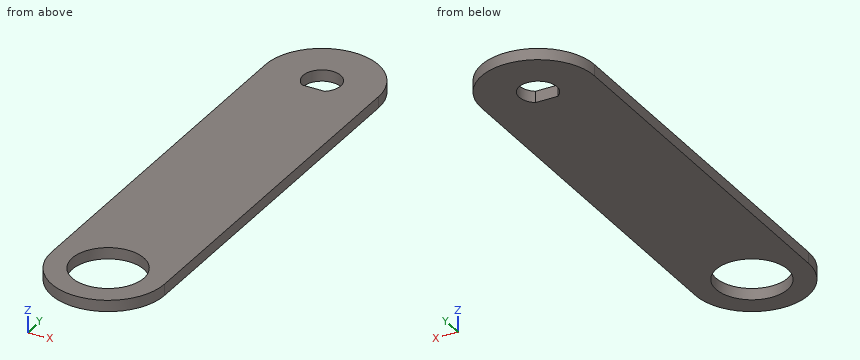
```python
from build123d import *

# Parameters (mm, degrees)
SKETCH_1_R      = 9.5
EXTRUDE_1_DEPTH = 3


with BuildPart() as part:
    # 草图1 → 凸台-拉伸1 (new body)
    with BuildSketch(Plane.XY):
        with BuildLine():
            Line((-15, 0), (-15, -100))
            ThreePointArc((-15, -100), (0, -115), (15, -100))
            Line((15, -100), (15, 0))
            ThreePointArc((15, 0), (0, 15), (-15, 0))
        make_face()
        with Locations((0, -100)):
            Circle(SKETCH_1_R, mode=Mode.SUBTRACT)
        with BuildLine():
            Line((0, -4), (3, -4))
            ThreePointArc((3, -4), (0, 5), (-3, -4))
            Line((-3, -4), (0, -4))
        make_face(mode=Mode.SUBTRACT)
    extrude(amount=EXTRUDE_1_DEPTH)


solid = part.part
```
The model under review builds one solid part; all positions refer to its coordinate system, in mm. Coordinates: 2 decimals unless noted, no trailing zeros. Order: outer loops, then holes, each group sorted by start corner. A loop starts at its lowest first (then second) coordinate and runs counter-clockwise, first axis right, second up. Notation, with made-up numbers: (85.25, 21) -> (117.25, 21) arc R17 ccw to (117.25, 29) -> close; hole circle Ø1 at (54, 2.25). An arc over 180 degrees is marked (long way). Answer in a Markdown table with one row per item. Add a question column.
Item 1: We need section C-C on x = -7. Write out the cut boundary in (y, z), plus the area to 3 significant figures.
Item 2: We need section A-A on z = 0.6. Write out the cut boundary in (x, y).
Item 3: We need section B-B on x = 0. Write out the cut boundary in (y, z).
Item 4: Clearance check with flat-ended pins moving along their axes: pin 1 (6 mm diameter, centred on x = 0, y = 0, fed in from -Z); pin 2 (0.9 mm diameter, centred on x = -1, z = 1.5, fed in from +Y). State where each tip first meets the part, or that it passes through.
Item 5: To check wall thickness, follow probe 1 along Y at (x, z) = (0, 0.65); probe 2 along Y at (x, z) = (-2, 2.75); probe 3 along X at (y, z) = (-3.5, 1.5). State the ranges of each line that lie inside material, in increasing order.
Final values:
| question | item | result |
|---|---|---|
| 1 | outline | (-113.27, 0) -> (-106.42, 0) -> (-106.42, 3) -> (-113.27, 3) -> close; (-93.58, 0) -> (13.27, 0) -> (13.27, 3) -> (-93.58, 3) -> close |
| 1 | area | 341 mm2 |
| 2 | outline | (-15, -100) arc R15 ccw to (15, -100) -> (15, 0) arc R15 ccw to (-15, 0) -> close; hole circle Ø19 at (0, -100); hole (-3, -4) -> (3, -4) arc R5 ccw (long way) to start |
| 3 | outline | (-115, 0) -> (-109.5, 0) -> (-109.5, 3) -> (-115, 3) -> close; (-90.5, 0) -> (-4, 0) -> (-4, 3) -> (-90.5, 3) -> close; (5, 0) -> (15, 0) -> (15, 3) -> (5, 3) -> close |
| 4 | pin 1 | passes through |
| 4 | pin 2 | stops at y = 14.99 |
| 5 | probe 1 | y = -115 to -109.5, -90.5 to -4, 5 to 15 |
| 5 | probe 2 | y = -114.87 to -109.29, -90.71 to -4, 4.58 to 14.87 |
| 5 | probe 3 | x = -15 to -3.57, 3.57 to 15 |
